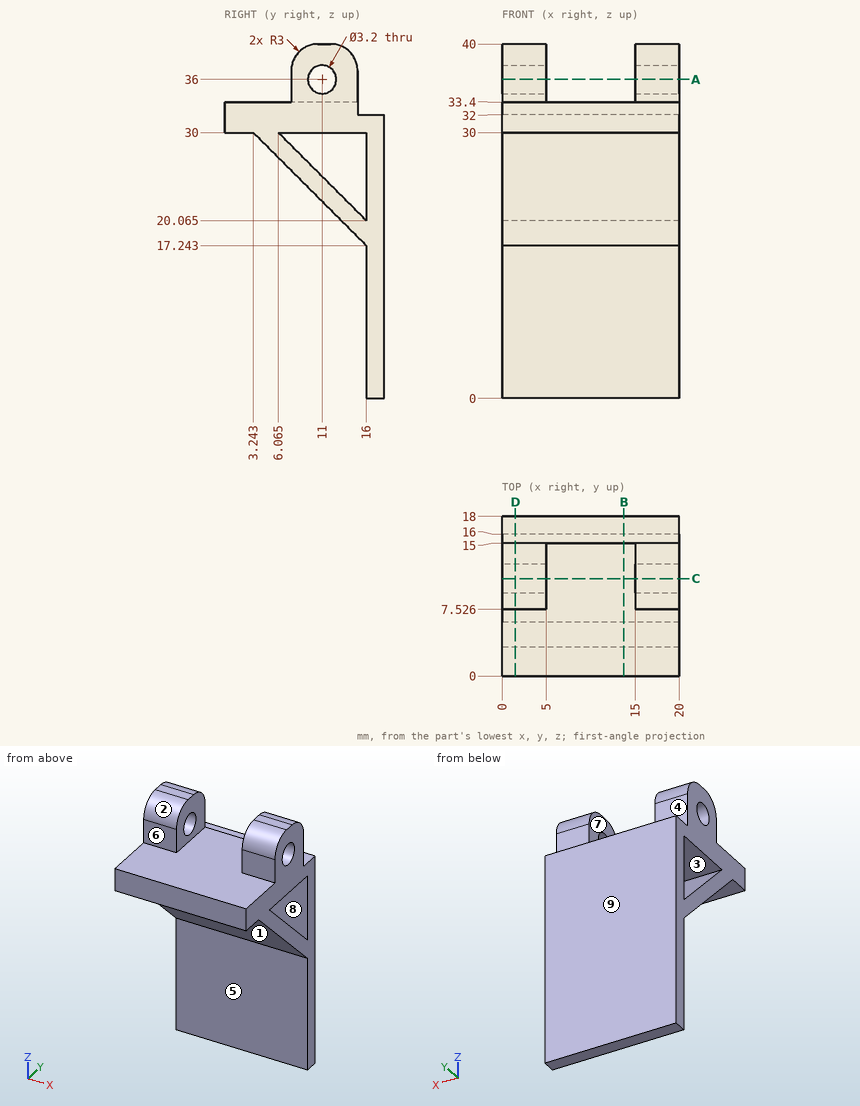
Design review of the part shown in the three views and the two pictorial views. Dimensions are in mm from the part's minimum x, y and z. A direction names the side the tool comes from. Round coordinates to 2 decimals unless told otherwise and drop trailing zeros. Loops run counter-clockwise (first coordinate to the right, second up) from the corner with the lowest first, then second, coordinate; pieces in that order, holes last.
1) Tool access review of the marked faces 5, 6, 7, 8 and 9: name each direction out of +Z, -Z, +X, -X, +Y, -Y from which nothing blocks a thin tool from reaching the whole face with its end or side.
Values follow:
face 5: -Z, +X, -X, -Y
face 6: +Z, +X, -X, -Y
face 7: +Z, +Y, -Y
face 8: +X, -X
face 9: +Z, -Z, +X, -X, +Y
2) Consider section A-A on z = 36. State the section outline as (x, y) points.
Values follow:
outline: (0, 7.53) - (5, 7.53) - (5, 9.4) - (0, 9.4) - close; (0, 12.6) - (5, 12.6) - (5, 15) - (0, 15) - close; (15, 7.53) - (20, 7.53) - (20, 9.4) - (15, 9.4) - close; (15, 12.6) - (20, 12.6) - (20, 15) - (15, 15) - close
3) The part is to be moulded in two halves that separate along Z. For the marked faces 1, 2, 3 and 4, say which applies: pulls with the +Z half, pulls with the -Z half, needs draft (parallel to the pull), parting line crosses it, or undercut.
Values follow:
face 1: pulls with the -Z half
face 2: pulls with the +Z half
face 3: undercut
face 4: needs draft
4) Wall thickness on line 1 along Z through (x, y) = (1.65, 11) (1 decimal); line 2 along X through (y, z) = (13.5, 38); line 3 along Z through (x, y) = (13.5, 2.75): over which ranges is each line inside the solid? List them lowest first.
Values follow:
line 1: z = 22.2 to 25.1, 30 to 34.4, 37.6 to 40
line 2: x = 0 to 5, 15 to 20
line 3: z = 30 to 33.4
5) Clearance check with flat-ended pins moving along their axes: P1, Ø3.5, axis at x = 12.5, y = 1, coming from the -Z side; P2, Ø10, axis at x = 8.5, z = 21.5, coming from the -Y side; P3, Ø3, axis at x = 5.5, y = 7, coming from the +Z side; P4, Ø1.9, axis at y = 11, z = 36, coming from the -X side. State where each tip first meets the part, or that it passes through.
Values follow:
P1: stops at z = 30
P2: stops at y = 6.74
P3: stops at z = 39.13
P4: passes through
6) Consider section D-D on x = 1.5. State the section outline as (y, z) points (1 decimal).
Values follow:
outline: (0, 30) - (3.2, 30) - (16, 17.2) - (16, 0) - (18, 0) - (18, 32) - (15, 32) - (15, 37) arc R3 ccw to (12, 40) - (10.5, 40) arc R3 ccw to (7.5, 37) - (7.5, 33.4) - (0, 33.4) - close; hole (6.1, 30) - (16, 20.1) - (16, 30) - close; hole circle Ø3.2 at (11, 36)
7) Consider section B-B on x = 13.75. State the section outline as (y, z) points (1 decimal), then the cut area to 3 significant figures.
Values follow:
outline: (0, 30) - (3.2, 30) - (16, 17.2) - (16, 0) - (18, 0) - (18, 32) - (15, 32) - (15, 33.4) - (0, 33.4) - close; hole (6.1, 30) - (16, 20.1) - (16, 30) - close
area: 149 mm2
8) Consider section C-C on y = 11. State the section outline as (x, z) points (1 decimal).
Values follow:
outline: (0, 22.2) - (20, 22.2) - (20, 25.1) - (0, 25.1) - close; (0, 30) - (20, 30) - (20, 34.4) - (15, 34.4) - (15, 33.4) - (5, 33.4) - (5, 34.4) - (0, 34.4) - close; (0, 37.6) - (5, 37.6) - (5, 40) - (0, 40) - close; (15, 37.6) - (20, 37.6) - (20, 40) - (15, 40) - close
